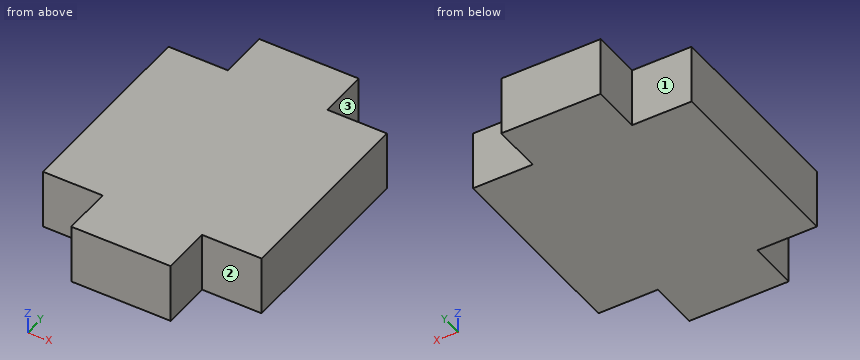
```python
from build123d import *

# Parameters (mm, degrees)
SKETCH_1_W      = 3
SKETCH_1_H      = 10
SKETCH_1_W_2    = 5
SKETCH_1_H_2    = 15
EXTRUDE_1_DEPTH = 3


with BuildPart() as part:
    # 草图1 → 凸台-拉伸1 (new body)
    with BuildSketch(Plane.XY):
        with Locations((-4, 0)):
            Rectangle(SKETCH_1_W, SKETCH_1_H)
        Rectangle(SKETCH_1_W_2, SKETCH_1_H_2)
        with Locations((4, 0)):
            Rectangle(SKETCH_1_W, SKETCH_1_H)
    extrude(amount=EXTRUDE_1_DEPTH)


solid = part.part
```
Here's how the part is built. I have some questions about the finished solid (model axes, mm). Face numbers are marked on the shaded views. A direction names the side the tool comes from. Coordinates: 2 decimals unless noted, no trailing zeros. Write each loop counter-clockwise with the first axis right and the second up, starting at its lowest first coordinate (ties: lowest second). Pieces come first, ordered by that corner, then holes. Notation, with made-up numbers: M 9.25,55 L 24.25,55 A18 ccw 24.25,76 Z; hole C -39,17 d2. An arc over 180 degrees is marked long. Answer as CSV lines item,"result". Start each with the question number.
Q1. I need wall thicknesses on probe 1 along X at (y, z) = (5.75, 1.4); probe 2 along Y at (x, z) = (-4.25, 1.3). Which ranges of each line are inside material? Lowest first, please. Write a range as [from, to].
Q2. Suppose I cut it at C-C, the plane x = -3.5. List the corners of the cut face in (y, z) for me.
Q3. Suppose I cut it at B-B, the plane y = 6.5. List the corners of the cut face in (x, z) for me.
Q4. For the marked faces 1, 2 and 3, which set-ups out of +Z, -Z, +X, -X, +Y, -Y let a thin tool reach every point of the face, with its end or its side?
Q5. Suppose I cut it at A-A, the plane z = 0.8. List the corners of the cut face in (x, y) for me.
Q6. Will this pin go through, and if not, where does the flat tip stop? pin 1 Ø1.5 at (x, z) = (4.5, 1) entering from +Y.
Entries:
1,probe 1,"x = [-2.5, 2.5]"
1,probe 2,"y = [-5, 5]"
2,outline,"M -5,0 L 5,0 L 5,3 L -5,3 Z"
3,outline,"M -2.5,0 L 2.5,0 L 2.5,3 L -2.5,3 Z"
4,face 1,"+Z, -Z, -X, +Y"
4,face 2,"+Z, -Z, +X, -Y"
4,face 3,"+Z, -Z, +X, +Y"
5,outline,"M -5.5,-5 L -2.5,-5 L -2.5,-7.5 L 2.5,-7.5 L 2.5,-5 L 5.5,-5 L 5.5,5 L 2.5,5 L 2.5,7.5 L -2.5,7.5 L -2.5,5 L -5.5,5 Z"
6,pin 1,"stops at y = 5"
